```python
from build123d import *

# Parameters (mm, degrees)
F0_R     = 5.5
F0_R_2   = 1.3
F1_DEPTH = 1.8


with BuildPart() as f1:
    # F0 (on Front) → F1 (new body)
    with BuildSketch(Plane.XZ):
        Circle(F0_R)
        with BuildLine():
            ThreePointArc((-0.75, 3.725252), (0, 3.8), (0.75, 3.725252))
            ThreePointArc((0.75, 3.725252), (2.940238, 2.407281), (3.8, 0))
            ThreePointArc((3.8, 0), (3.787062, -0.313306), (3.748337, -0.624478))
            ThreePointArc((3.748337, -0.624478), (3.550562, -1.354072), (3.212284, -2.030082))
            ThreePointArc((3.212284, -2.030082), (0, -3.8), (-3.212284, -2.030082))
            ThreePointArc((-3.212284, -2.030082), (-3.550562, -1.354072), (-3.748337, -0.624478))
            ThreePointArc((-3.748337, -0.624478), (-3.128705, 2.156665), (-0.75, 3.725252))
        make_face(mode=Mode.SUBTRACT)
        with BuildLine():
            Line((3.748337, -0.624478), (2.499741, -0.036019))
            ThreePointArc((2.499741, -0.036019), (2.372029, -0.789606), (2.022598, -1.469387))
            Line((2.022598, -1.469387), (3.212284, -2.030082))
            ThreePointArc((3.212284, -2.030082), (3.550562, -1.354072), (3.748337, -0.624478))
        make_face()
        with BuildLine():
            ThreePointArc((-0.75, 2.384848), (0, 2.5), (0.75, 2.384848))
            Line((0.75, 2.384848), (0.75, 3.725252))
            ThreePointArc((0.75, 3.725252), (0, 3.8), (-0.75, 3.725252))
            Line((-0.75, 3.725252), (-0.75, 2.384848))
        make_face()
        with BuildLine():
            ThreePointArc((-2.022598, -1.469387), (-2.372029, -0.789606), (-2.499741, -0.036019))
            Line((-2.499741, -0.036019), (-3.748337, -0.624478))
            ThreePointArc((-3.748337, -0.624478), (-3.550562, -1.354072), (-3.212284, -2.030082))
            Line((-3.212284, -2.030082), (-2.022598, -1.469387))
        make_face()
        with BuildLine():
            ThreePointArc((2.499741, -0.036019), (2.499935, -0.01801), (2.5, 0))
            ThreePointArc((2.5, 0), (2.015564, 1.47902), (0.75, 2.384848))
            ThreePointArc((0.75, 2.384848), (0, 2.5), (-0.75, 2.384848))
            ThreePointArc((-0.75, 2.384848), (-2.026167, 1.464462), (-2.499741, -0.036019))
            ThreePointArc((-2.499741, -0.036019), (-2.372029, -0.789606), (-2.022598, -1.469387))
            ThreePointArc((-2.022598, -1.469387), (0, -2.5), (2.022598, -1.469387))
            ThreePointArc((2.022598, -1.469387), (2.372029, -0.789606), (2.499741, -0.036019))
        make_face()
        Circle(F0_R_2, mode=Mode.SUBTRACT)
    extrude(amount=F1_DEPTH)


solid = f1.part
```
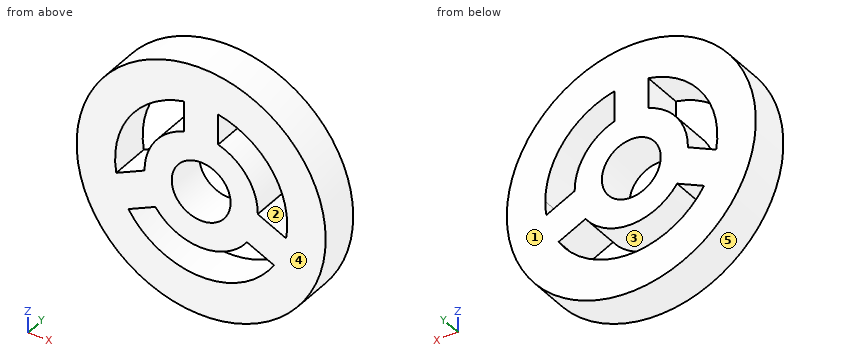
Source: CAD feature listing. Evaluate the final solid. Frame: model axes, mm. Face numbers are marked on the shaded views. A direction names the side the tool comes from. Give positions to 0.01 mm unless a question says otherwise; leave off trailing zeros. Loops run counter-clockwise (first coordinate to the right, second up) from the corner with the lowest first, then second, coordinate; pieces in that order, holes last. Notation, with made-up numbers: M -8,70.25 L -1,70.25 A14 cw -1,80.25 Z; hole C -6.5,13.5 d1. An arc over 180 degrees is marked long. Put each result on its own line as item: value.
Q1. Section C-C (x = -2.25). Return the cut outline in (y, z), and give its area (3 significant figures).
Response values:
outline: M -1.8,-5.02 L 0,-5.02 L 0,-3.06 L -1.8,-3.06 Z; M -1.8,-1.58 L 0,-1.58 L 0,1.09 L -1.8,1.09 Z; M -1.8,3.06 L 0,3.06 L 0,5.02 L -1.8,5.02 Z
area: 11.8 mm²
Q2. Section B-B (y = -1). Count the separate pieces of the cut face and the enclosed holes in it, and give its area (3 significant figures).
Response values:
separate pieces: 1
enclosed holes: 4
area: 69.9 mm²
Q3. Reachability of the marked faces 1 and 2 from +Z, -Z, +X, -X, +Y, -Y: full face, straight path, thin tool, end or side. Return the list, or none.
Response values:
face 1: +Z, -Z, +X, -X, +Y
face 2: +Y, -Y
Q4. Section A-A (x = 0). Return the cut outline in (y, z), and give its area (3 significant figures).
Response values:
outline: M -1.8,-5.5 L 0,-5.5 L 0,-3.8 L -1.8,-3.8 Z; M -1.8,-2.5 L 0,-2.5 L 0,-1.3 L -1.8,-1.3 Z; M -1.8,1.3 L 0,1.3 L 0,5.5 L -1.8,5.5 Z
area: 12.8 mm²
Q5. Section D-D (x = -4). Return the cut outline in (y, z).
Response values:
outline: M -1.8,-3.77 L 0,-3.77 L 0,3.77 L -1.8,3.77 Z
Q6. Mould query, pull axis X, two halves, no side actions, for the marked faces 3, 4 and 5. Classes: released by +X, released by -X, zero draft, split by the parting line, or undercut.
Response values:
face 3: undercut
face 4: zero draft
face 5: split by the parting line
Q7. Line query: probe 1 along Z at (x, y) = (0, -0.85); probe 2 along Z at (x, y) = (-0.5, -1.7); probe 3 along X at (y, z) = (-1.7, 3). Output: solid intervals per line, ascending. Write a range as [from, to].
Response values:
probe 1: z = [-5.5, -3.8], [-2.5, -1.3], [1.3, 5.5]
probe 2: z = [-5.48, -3.77], [-2.45, -1.2], [1.2, 5.48]
probe 3: x = [-4.61, -2.33], [-0.75, 0.75], [2.33, 4.61]
